```python
from build123d import *

# Parameters (mm, degrees)
SKETCH3_R             = 21.5
BOSS_EXTRUDE3_DEPTH   = 1
SKETCH10_R            = 1.1
SKETCH10_W            = 22.5
SKETCH10_H            = 12.2
CUT_EXTRUDE3_DEPTH    = 170.731914631
F_6_CLEARANCE_HOLE1_D = 3.7973


with BuildPart() as part:
    # Sketch3 → Boss-Extrude3 (new body)
    with BuildSketch(Plane(origin=(0, 0, 0), x_dir=(1, 0, 0), z_dir=(0, 1, 0))):
        with BuildLine():
            Line((-132.226234517, -18.972612677), (132.537224892, -18.972612677))
            Line((132.537224892, -18.972612677), (132.537224892, 26.561617598))
            ThreePointArc((132.537224892, 26.561617598), (0.155495187, 106.027387323), (-132.226234517, 26.561617598))
            Line((-132.226234517, 26.561617598), (-132.226234517, -18.972612677))
        make_face()
        with Locations(Location((-96.926544138, 26.561617598, 0), (0, 0, 270))):
            Circle(SKETCH3_R, mode=Mode.SUBTRACT)
        with Locations(Location((97.237534512, 26.561617598, 0), (0, 0, 270))):
            Circle(SKETCH3_R, mode=Mode.SUBTRACT)
        with Locations(Location((-36.926544138, 70.154169278, 0), (0, 0, 270))):
            Circle(SKETCH3_R, mode=Mode.SUBTRACT)
        with Locations(Location((37.237534512, 70.154169278, 0), (0, 0, 270))):
            Circle(SKETCH3_R, mode=Mode.SUBTRACT)
    extrude(amount=BOSS_EXTRUDE3_DEPTH)

    # Sketch10 → Cut-Extrude3 (cut, through all)
    with BuildSketch(Plane(origin=(0, 0, 0), x_dir=(-1, 0, 0), z_dir=(0, -1, 0))):
        with Locations(Location((-31.076423082, 23.72316033, 0), (0, 0, 90))):
            Circle(SKETCH10_R)
        with Locations(Location((-3.276423082, 23.72316033, 0), (0, 0, 90))):
            Circle(SKETCH10_R)
        with Locations((-17.176423082, 23.72316033)):
            Rectangle(SKETCH10_W, SKETCH10_H)
    extrude(amount=-CUT_EXTRUDE3_DEPTH, mode=Mode.SUBTRACT)

    # #6 Clearance Hole1 (through all)
    with Locations(Plane(origin=(0, 0, 0), x_dir=(-1, 0, 0), z_dir=(0, -1, 0))):
        with Locations((-97.237534512, 56.561617598), (-67.237534512, 26.561617598), (-67.237534512, 70.154169278), (-7.237534512, 70.154169278), (6.926544138, 70.154169278), (66.926544138, 70.154169278), (96.926544138, 56.561617598), (66.926544138, 26.561617598), (19.154347381, 19.79486368), (45.291365084, 8.12316033), (33.361365084, 8.12316033), (6.061135322, 96.611330123), (-5.86886721, 96.611330123), (25.648240263, 24.024740184)):
            Hole(F_6_CLEARANCE_HOLE1_D / 2)


solid = part.part
```
Work out the finished part from the listing and answer in its coordinate system (mm). Round coordinates to 2 decimals unless told otherwise and drop trailing zeros. Loops run counter-clockwise (first coordinate to the right, second up) from the corner with the lowest first, then second, coordinate; pieces in that order, holes last. Notation, with made-up numbers: M 82.25,69 L 100.25,69 A26 cw 100.25,95 Z; hole C 31.5,1.25 d9. An arc over 180 degrees is marked long. Use CSV: the item, a comma, the result in double quotes.
Q1. Consider L1, parallel to Z at x = 97, y = 0.7; L2, parallel to X at y = 0.55, z = -34; L3, parallel to X at y = 0.5, z = -63. Determine where each line is inside the solid, lowest interval first.
Determined:
L1,"-70.57 to -58.45, -54.68 to -48.06, -5.06 to 18.97"
L2,"-127.99 to -117.1, -76.75 to 77.07, 117.41 to 128.3"
L3,"-105 to -57.2, -16.65 to 16.96, 57.51 to 105.31"
Q2. Section D-D, the plane z = -12.5 is taken. Determine the outline of the cut face in (x, y), then the cut area to 3 significant figures.
Determined:
outline,"M -132.23,0 L -113.19,0 L -113.19,1 L -132.23,1 Z; M -80.66,0 L 80.97,0 L 80.97,1 L -80.66,1 Z; M 113.5,0 L 132.54,0 L 132.54,1 L 113.5,1 Z"
area,"200 mm2"
Q3. Section A-A, the plane z = -64 is taken. Determine the outline of the cut face in (x, y), then the cut area to 3 significant figures.
Determined:
outline,"M -103.97,0 L -57.53,0 L -57.53,1 L -103.97,1 Z; M -16.33,0 L 16.64,0 L 16.64,1 L -16.33,1 Z; M 57.84,0 L 104.28,0 L 104.28,1 L 57.84,1 Z"
area,"126 mm2"
Q4. Section B-B, the plane x = -102.5 is taken. Determine the outline of the cut face in (y, z).
Determined:
outline,"M 0,-65.4 L 1,-65.4 L 1,-47.33 L 0,-47.33 Z; M 0,-5.8 L 1,-5.8 L 1,18.97 L 0,18.97 Z"
Q5. This flat-tipped pin is pushed along its axis until it touches: pin 1 (3 mm diameter, centred on x = 3.28, z = -23.72, fed in from +Y). Where does it stop, or does it pass through?
Determined:
pin 1,"y = 1"
Q6. Section C-C, the plane y = 0.85 is taken. State how many separate pieces and enclosed holes the cut face has, then the cut area to 3 significant figures.
Determined:
separate pieces,"1"
enclosed holes,"21"
area,"20,800 mm2"
Q7. The mould has two halves that part along X. Classify faces 1 (the flat face through (-2, 1, -31)), 2 (the cylindrical face through (51.77, 0.49, -86)), 3 (the cylindrical face through (2.43, 0.49, -106.01)): pulls with the +X half, pulls with the -X half, needs draft (parallel to the pull), parting line crosses it, or undercut.
Determined:
face 1,"needs draft"
face 2,"undercut"
face 3,"parting line crosses it"
